```python
from build123d import *

# Parameters (mm, degrees)
SM_BASE_FLANGE_1_DEPTH   = 60
CUT_EXTRUDE_1_DEPTH      = 158.919093209
CUT_EXTRUDE_1_DEPTH_BACK = 158.919093209
FILLET_1_R               = 5
SM_EDGE_FLANGE_1_DEPTH   = 134.6
HOLE_WIZARD_6_1_6_1_1_D  = 6.1
HOLE_WIZARD_3_0_3_1_D    = 3
CUT_EXTRUDE_2_DEPTH      = 10
HOLE_WIZARD_4_0_4_1_D    = 4
FILLET_2_R               = 3


# Sheet-metal steps are written as plain solids
with BuildPart() as part:
    # Sketch 1 → Базовая кромка1 (new, symmetric)
    with BuildSketch(Plane.XY):
        with BuildLine():
            Line((-85, 0), (-71.5, 0))
            ThreePointArc((-71.5, 0), (-70.439339828, 0.439339828), (-70, 1.5))
            Line((-70, 1.5), (-70, 116.1))
            ThreePointArc((-70, 116.1), (-69.209188309, 118.009188309), (-67.3, 118.8))
            Line((-67.3, 118.8), (67.3, 118.8))
            ThreePointArc((67.3, 118.8), (69.209188309, 118.009188309), (70, 116.1))
            Line((70, 116.1), (70, 1.5))
            ThreePointArc((70, 1.5), (70.439339828, 0.439339828), (71.5, 0))
            Line((71.5, 0), (85, 0))
            Line((85, 0), (85, -1.2))
            Line((85, -1.2), (71.5, -1.2))
            ThreePointArc((71.5, -1.2), (69.590811691, -0.409188309), (68.8, 1.5))
            Line((68.8, 1.5), (68.8, 116.1))
            ThreePointArc((68.8, 116.1), (68.360660172, 117.160660172), (67.3, 117.6))
            Line((67.3, 117.6), (-67.3, 117.6))
            ThreePointArc((-67.3, 117.6), (-68.360660172, 117.160660172), (-68.8, 116.1))
            Line((-68.8, 116.1), (-68.8, 1.5))
            ThreePointArc((-68.8, 1.5), (-69.590811691, -0.409188309), (-71.5, -1.2))
            Line((-71.5, -1.2), (-85, -1.2))
            Line((-85, -1.2), (-85, 0))
        make_face()
    extrude(amount=SM_BASE_FLANGE_1_DEPTH, both=True)

    # Эскиз6 → Вырез-Вытянуть1 (cut, two sides: drawn at the far end of the back side and taken through both)
    with BuildSketch(Plane(origin=(0, 0, 0), x_dir=(0, 0, -1), z_dir=(1, 0, 0)).offset(-CUT_EXTRUDE_1_DEPTH_BACK)):
        Polygon((-60, 28.8), (-20, 108.8), (-20, 118.8), (-60, 118.8), align=None)
        Polygon((60, 108.8), (20, 28.8), (20, -1.2), (60, -1.2), align=None)
    extrude(amount=CUT_EXTRUDE_1_DEPTH + CUT_EXTRUDE_1_DEPTH_BACK, mode=Mode.SUBTRACT)

    # Скругление1
    fillet_1_edges = [part.edges().sort_by_distance(p)[0] for p in [
        (-69.4, 108.8, -60),
        (-69.4, 28.8, -20),
        (-85, -0.6, -20),
        (69.4, 108.8, -60),
        (69.4, 28.8, -20),
        (85, -0.6, -20),
        (69.4, 28.8, 60),
        (69.4, 108.8, 20),
        (-69.4, 28.8, 60),
        (-69.4, 108.8, 20),
        (-85, -0.6, 60),
        (85, -0.6, 60),
    ]]
    fillet(fillet_1_edges, radius=FILLET_1_R)

    # Ребро-кромка1 section (across the edge) → Ребро-кромка1 (add)
    with BuildSketch(Plane(origin=(-67.3, 117.6, -61.5), x_dir=(0, 0, 1), z_dir=(1, 0, 0))):
        with BuildLine():
            Line((-1.2, 1.5), (-1.2, 8.8))
            Line((-1.2, 8.8), (0, 8.8))
            Line((0, 8.8), (0, 1.5))
            ThreePointArc((0, 1.5), (0.439339828, 0.439339828), (1.5, 0))
            Line((1.5, 0), (1.5, -1.2))
            ThreePointArc((1.5, -1.2), (-0.409188309, -0.409188309), (-1.2, 1.5))
        make_face()
    extrude(amount=SM_EDGE_FLANGE_1_DEPTH)

    # Диаметр отверстия Ø6.1 (6.1)1 (through all)
    with Locations(Plane(origin=(0, 0, 0), x_dir=(1, 0, 0), z_dir=(0, 1, 0))):
        with Locations((-78, 13), (-78, -53), (78, -53), (78, 13)):
            Hole(HOLE_WIZARD_6_1_6_1_1_D / 2)

    # Диаметр отверстия Ø3.0 (3)1 (through all)
    with Locations(Plane(origin=(0, 117.6, 0), x_dir=(-1, 0, 0), z_dir=(0, -1, 0))):
        with Locations((-20, -14), (-28, 56), (28, 56), (20, -14)):
            Hole(HOLE_WIZARD_3_0_3_1_D / 2)

    # Эскиз14 → Вырез-Вытянуть2 (cut)
    with BuildSketch(Plane.XZ.offset(-117.6)):
        with BuildLine():
            Line((-9.1, -8), (-45.1, -8))
            ThreePointArc((-45.1, -8), (-46.514213562, -8.585786438), (-47.1, -10))
            Line((-47.1, -10), (-47.1, -46))
            ThreePointArc((-47.1, -46), (-46.514213562, -47.414213562), (-45.1, -48))
            Line((-45.1, -48), (-9.1, -48))
            ThreePointArc((-9.1, -48), (-7.685786438, -47.414213562), (-7.1, -46))
            Line((-7.1, -46), (-7.1, -10))
            ThreePointArc((-7.1, -10), (-7.685786438, -8.585786438), (-9.1, -8))
        make_face()
    extrude(amount=-CUT_EXTRUDE_2_DEPTH, mode=Mode.SUBTRACT)

    # Диаметр отверстия Ø4.0 (4)1 (through all)
    with Locations(Plane(origin=(70, 0, 0), x_dir=(0, 0, -1), z_dir=(1, 0, 0))):
        with Locations((-12.819660113, 100.8), (44.819660113, 100.8), (26.931116293, 65.02291236), (-30.708203932, 65.02291236), (-48.596747752, 29.24582472), (9.042572473, 29.24582472)):
            Hole(HOLE_WIZARD_4_0_4_1_D / 2)

    # Скругление2
    fillet_2_edges = [part.edges().sort_by_distance(p)[0] for p in [
        (-67.3, 108.8, -62.1),
        (67.3, 108.8, -62.1),
    ]]
    fillet(fillet_2_edges, radius=FILLET_2_R)


solid = part.part
```
Model file for the job. Use its own axes, mm. A direction names the side the tool comes from. Give positions to 0.01 mm unless a question says otherwise; leave off trailing zeros. Order: outer loops, then holes, each group sorted by start corner. A loop starts at its lowest first (then second) coordinate and runs counter-clockwise, first axis right, second up.
1) Saw through at A-A, the plane z = -13. Count the separate pieces of the cut face and the enclosed holes in it, then the cut area to 3 significant figures.
2) Wall check: probe 1 along Z at (x, y) = (78, -0.9); probe 2 along X at (y, z) = (24, 20); probe 3 along Z at (x, y) = (-20, 118.2). Give the ranges that are in metal, low to high.
3) 3-axis set-ups, long thin cutter, end or side, ignore diameter. For faces 4 (the flat face through (69.8, 10.1, -20)), 5 (the flat face through (-1, 112, -61.5)), 6 (the cylindrical face through (-69.41, 31.23, -9.3)): which of +Z, -Z, +X, -X, +Y, -Y reach the whole face in a straight line?
4) Saw through at C-C, the plane z = 43. Write the cut outline in (x, y), then the cut area to 3 significant figures.
5) Saw through at D-D, the plane x = -24.5. Write the cut outline in (y, z), then the cut area to 3 significant figures.
6) Pin check, flat tips, straight feed: pin 1 (4.5 mm diameter, centred on y = 29.25, z = -9.04, fed in from +X); pin 2 (5 mm diameter, centred on x = 20, z = 14, fed in from -Y); pin 3 (11 mm diameter, centred on x = 77, z = 8, fed in from +Y); pin 4 (3 mm diameter, centred on y = 65.02, z = -26.93, fed in from +X). Stop position of each tip, or through.
7) Mould opens along X. For faces 1 (the cylindrical face through (80.42, -0.608, 54.856)), 2 (the cylindrical face through (69.39, 66.37, -28.41)), 3 (the cylindrical face through (-75.58, -0.608, 54.856)) say: +X half, -X half, draft (parallel to the pull), parting line (faces both ways), or undercut.
8) Saw through at B-B, the plane y = 89. Write the cut outline in (x, z).
Computed:
1. separate pieces: 4
1. enclosed holes: 0
1. area: 422 mm2
2. probe 1: z = -20 to -16.05, -9.95 to 49.95, 56.05 to 60
2. probe 2: x = -70 to -68.8, 68.8 to 70
2. probe 3: z = -61.7 to -48, -8 to 12.5, 15.5 to 20
3. face 4: -Z, +X, -X, -Y
3. face 5: +Z, +X, -X, -Y
3. face 6: +X, -X
4. outline: (-85, -1.2) - (-71.5, -1.2) arc R2.7 ccw to (-68.8, 1.5) - (-68.8, 62.8) - (-70, 62.8) - (-70, 1.5) arc R1.5 cw to (-71.5, 0) - (-85, 0) - close; (68.8, 1.5) arc R2.7 ccw to (71.5, -1.2) - (85, -1.2) - (85, 0) - (71.5, 0) arc R1.5 cw to (70, 1.5) - (70, 62.8) - (68.8, 62.8) - close
4. area: 187 mm2
5. outline: (108.8, -62.7) - (116.1, -62.7) arc R2.7 ccw to (118.8, -60) - (118.8, -48) - (117.6, -48) - (117.6, -60) arc R1.5 cw to (116.1, -61.5) - (108.8, -61.5) - close; (117.6, -8) - (118.8, -8) - (118.8, 20) - (117.6, 20) - close
5. area: 60.7 mm2
6. pin 1: stops at x = 70
6. pin 2: stops at y = 117.6
6. pin 3: stops at y = 0
6. pin 4: passes through
7. face 1: undercut
7. face 2: draft
7. face 3: undercut
8. outline: (-70, -50.1) - (-68.8, -50.1) - (-68.8, 29.9) - (-70, 29.9) - close; (68.8, -50.1) - (70, -50.1) - (70, 29.9) - (68.8, 29.9) - close
